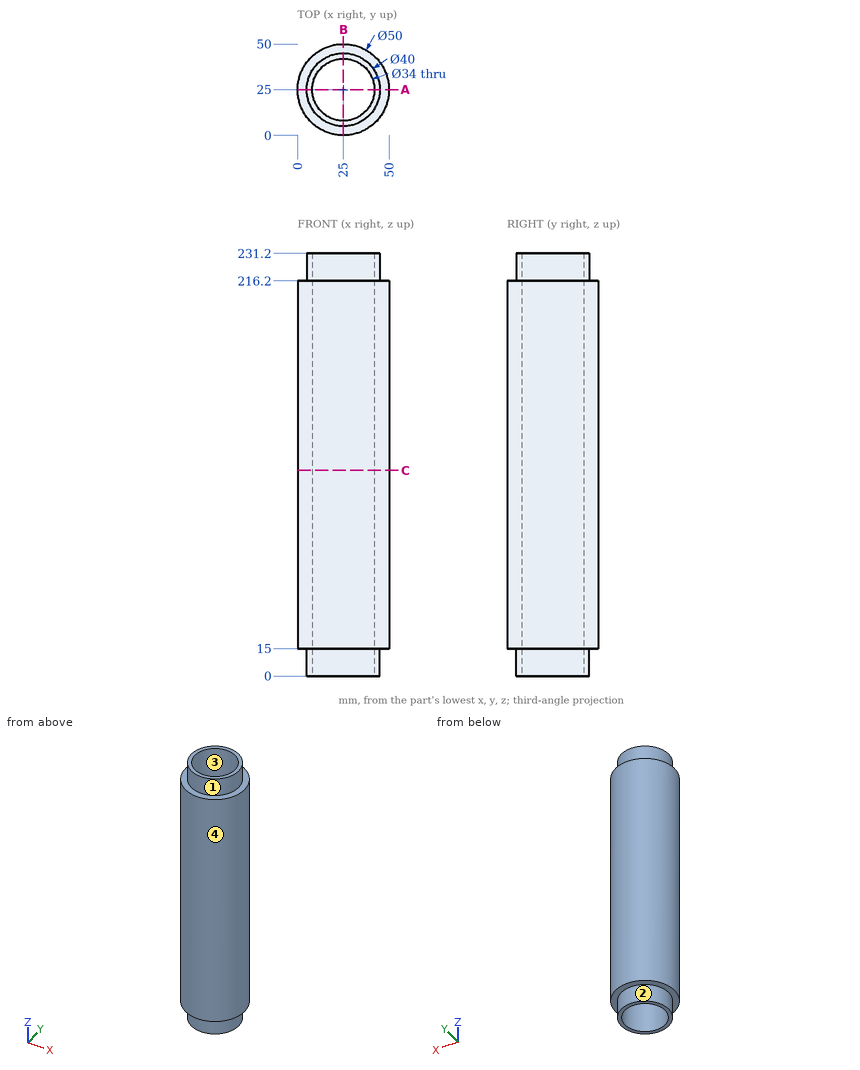
Job drawing, mm, ordinate dimensions from the low corner. One solid piece. A direction names the side the tool comes from. Coordinates: 2 decimals unless noted, no trailing zeros. Loops run counter-clockwise (first coordinate to the right, second up) from the corner with the lowest first, then second, coordinate; pieces in that order, holes last. Notation, with made-up numbers: (29, 87) -> (70, 87) arc R25 cw to (70, 100) -> close; hole circle Ø4 at (13.25, 67.25). An arc over 180 degrees is marked (long way). One line per item, written item: value.
1. Slice it at C-C on z = 112.5. Write the cut outline in (x, y), and give its area (3 significant figures).
Answers:
outline: circle Ø50 at (25, 25); hole circle Ø34 at (25, 25)
area: 1,060 mm^2
2. Which spindle directions (+Z, -Z, +X, -X, +Y, -Y) get a long thin tool onto all of the face, cutting with end or side? Do the marked faces 1 and 2. Say none if no direction does.
Answers:
face 1: +Z
face 2: -Z
3. Flat gauge pins, fed straight in: P1, Ø3, axis at x = 6, z = 75.5, coming from the +Y side; P2, Ø15, axis at x = 30, y = 30.5, coming from the -Z side; P3, Ø1.5, axis at x = 33, z = 154.5, coming from the -Y side; P4, Ø8, axis at y = 31, z = 177, coming from the +X side. Where does each tip first touch, or does it go through?
Answers:
P1: stops at y = 42.85
P2: passes through
P3: stops at y = 1.07
P4: stops at x = 49.92
4. Drill centre lines: line 1 (X direction, y = 24, z = 168.5); line 2 (Y direction, x = 25, z = 137); line 3 (Y direction, x = 36, z = 138.5). Where is each one in solid material? Low to high. Write a range as [from, to].
Answers:
line 1: x = [0.02, 8.03], [41.97, 49.98]
line 2: y = [0, 8], [42, 50]
line 3: y = [2.55, 12.04], [37.96, 47.45]
5. Pull direction X, two halves, no side cores. Call the marked faces 3 and 4: pulls with the +X half, pulls with the -X half, needs draft (parallel to the pull), parting line crosses it, or undercut.
Answers:
face 3: undercut
face 4: parting line crosses it
6. Slice it at A-A on y = 25. Write the cut outline in (x, z), and give its area (3 significant figures).
Answers:
outline: (0, 15) -> (5, 15) -> (5, 0) -> (8, 0) -> (8, 231.2) -> (5, 231.2) -> (5, 216.2) -> (0, 216.2) -> close; (42, 0) -> (45, 0) -> (45, 15) -> (50, 15) -> (50, 216.2) -> (45, 216.2) -> (45, 231.2) -> (42, 231.2) -> close
area: 3,400 mm^2
